Work out the finished part from the listing and answer in its coordinate system (mm). A direction names the side the tool comes from. Coordinates: 2 decimals unless noted, no trailing zeros. Write each loop counter-clockwise with the first axis right and the second up, starting at its lowest first coordinate (ties: lowest second). Pieces come first, ordered by that corner, then holes. Notation, with made-up numbers: M 71.5,7 L 89.5,7 A20 cw 89.5,27 Z; hole C -23,20 d9. An arc over 180 degrees is marked long. Use CSV: the item, a comma, the result in double quotes.
from build123d import *

# Parameters (mm, degrees)
SKETCH1_R           = 4.05
BOSS_EXTRUDE1_DEPTH = 40
SKETCH2_W           = 45.127997656
SKETCH2_H           = 26.248845412
BOSS_EXTRUDE2_DEPTH = 3


with BuildPart() as part:
    # Sketch1 → Boss-Extrude1 (new body)
    with BuildSketch(Plane(origin=(0, 0, 0), x_dir=(1, 0, 0), z_dir=(0, 1, 0))):
        Circle(SKETCH1_R)
    extrude(amount=BOSS_EXTRUDE1_DEPTH)

    # Sketch2 → Boss-Extrude2 (add)
    with BuildSketch(Plane.XZ):
        Rectangle(SKETCH2_W, SKETCH2_H)
    extrude(amount=BOSS_EXTRUDE2_DEPTH)


solid = part.part
Item 1: The part is cut by section A-A (x = 0). Write down the section's boundary in (y, z), then the cut area to 3 significant figures.
Answer:
outline,"M -3,-13.12 L 0,-13.12 L 0,-4.05 L 40,-4.05 L 40,4.05 L 0,4.05 L 0,13.12 L -3,13.12 Z"
area,"403 mm2"
Item 2: A tool of negligible diameter and unlimited length cuts with its end or side. For faces 1 (the face through (-0.878, 19.72, 3.954)), 2 (the face through (0, -1, 13.124)), from which of +Z, -Z, +X, -X, +Y, -Y can it reach the whole face along a straight path? Write none if from no direction.
Answer:
face 1,"+Y"
face 2,"+Z, +X, -X, +Y, -Y"
Item 3: Consider probe 1 along Y at (x, z) = (-9.5, -5.75); probe 2 along X at (y, z) = (17, -2); probe 3 along X at (y, z) = (12, 2.75). Determine where each line is inside the solid, lowest interval first.
Answer:
probe 1,"y = -3 to 0"
probe 2,"x = -3.52 to 3.52"
probe 3,"x = -2.97 to 2.97"
Item 4: Given pin 1 (12 mm diameter, centred on x = 0.5, y = 17, fed in from +Z); pin 2 (6 mm diameter, centred on y = 10, z = -2.5, fed in from -X); pin 3 (8 mm diameter, centred on y = 20, z = 2.5, fed in from +X), each flat-ended and moving along its own axis, determine where each tip first touches the part or whether it passes through.
Answer:
pin 1,"stops at z = 4.05"
pin 2,"stops at x = -4.05"
pin 3,"stops at x = 4.05"
Item 5: The part is cut by section D-D (x = -15). Write down the section's boundary in (y, z).
Answer:
outline,"M -3,-13.12 L 0,-13.12 L 0,13.12 L -3,13.12 Z"
Item 6: The part is cut by section B-B (z = 0). Write down the section's boundary in (x, y), then the cut area to 3 significant figures.
Answer:
outline,"M -22.56,-3 L 22.56,-3 L 22.56,0 L 4.05,0 L 4.05,40 L -4.05,40 L -4.05,0 L -22.56,0 Z"
area,"459 mm2"
Item 7: The part is cut by section C-C (y = 6). Write down the section's boundary in (x, z), then the cut area to 3 significant figures.
Answer:
outline,"C 0,0 d8.1"
area,"51.5 mm2"
